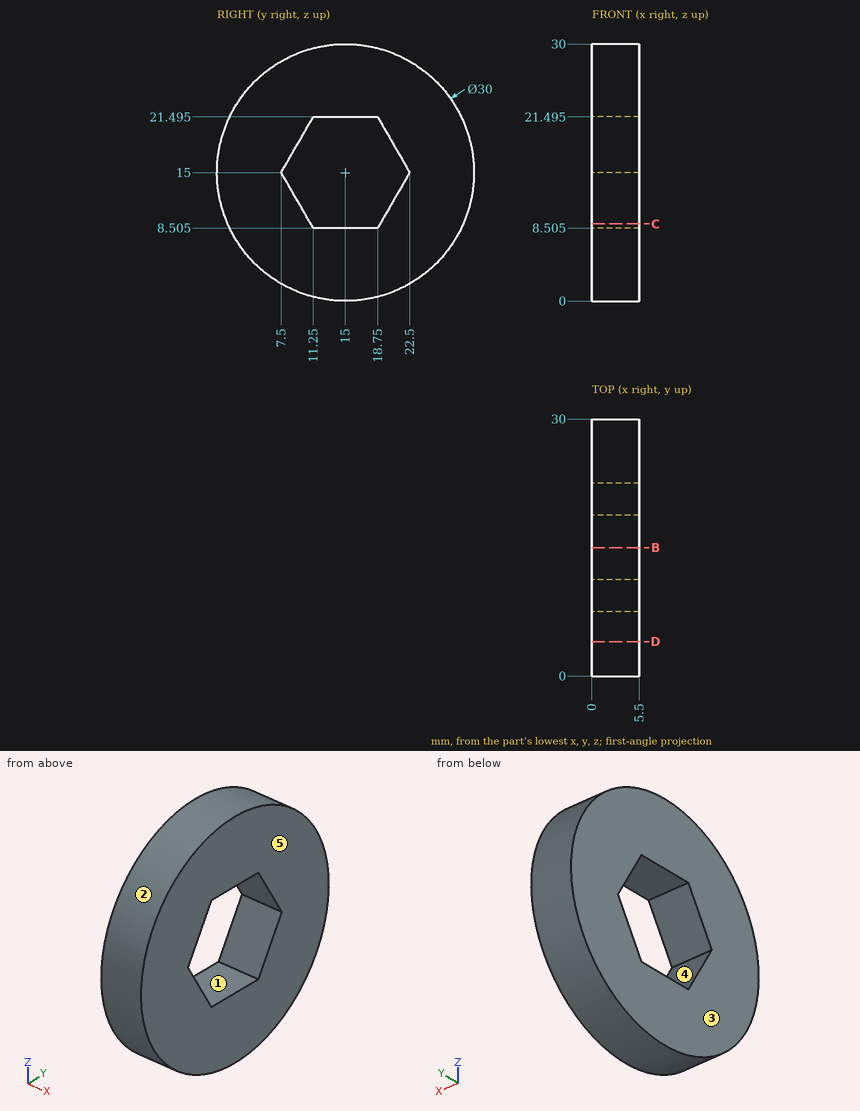
Here's the drawing with two shaded views (mm, measured from the low corner). I have some questions. A direction names the side the tool comes from. Give positions to 0.01 mm unless a question says otherwise; leave off trailing zeros. Order: outer loops, then holes, each group sorted by start corner. A loop starts at its lowest first (then second) coordinate and runs counter-clockwise, first axis right, second up. Notation, with made-up numbers: (29.25, -11.75) - (87.25, -11.75) arc R20 ccw to (87.25, 2.25) - close; hole circle Ø5 at (15.5, 59.5). An arc over 180 degrees is marked (long way). Use a Markdown table: item, result. Add a question column.
Q1. I'm going to push flat-ended pins straight in: pin 1 (2 mm diameter, centred on x = 1, y = 13.5, fed in from +Z); pin 2 (1 mm diameter, centred on x = 1, y = 23, fed in from -Z); pin 3 (2 mm diameter, centred on x = 3, y = 17.5, fed in from +Z) (3 decimals); pin 4 (1.5 mm diameter, centred on y = 18, z = 12, fed in from -X). Where does each tip first touch, or does it pass through?
Q2. If we section it at D-D on y = 4: Write out the boundary of the cut face in (x, z), plus the area to 3 significant figures.
Q3. Please list where these lines run through material, in increasing order: line 1 along Z through (x, y) = (1.65, 12.75) (1 decimal); line 2 along Z through (x, y) = (1.2, 11); line 3 along Y through (x, z) = (2.8, 17.25).
Q4. If we section it at B-B on y = 15: Write out the boundary of the cut face in (x, z) (1 decimal).
Q5. If we section it at C-C on z = 9: Write out the boundary of the cut face in (x, y), plus the area to 3 significant figures.
Q6. On a 3-axis mill with a long thin cutter (end or side, diameter ignored), from which of +Z, -Z, +X, -X, +Y, -Y can I reach the whole of each face in a straight line? I mean the marked faces 4 and 5. Say none if no direction works.
Q7. If we mould it in two halves opening along Z, with no side actions, what happens to the marked faces 1, 2 and 3? For each: released by +Z, released by -Z, zero draft, split by the parting line, or undercut.
Answers follow:
| question | item | result |
|---|---|---|
| 1 | pin 1 | stops at z = 29.99 |
| 1 | pin 2 | stops at z = 2.01 |
| 1 | pin 3 | stops at z = 29.925 |
| 1 | pin 4 | passes through |
| 2 | outline | (0, 4.8) - (5.5, 4.8) - (5.5, 25.2) - (0, 25.2) - close |
| 2 | area | 112 mm^2 |
| 3 | line 1 | z = 0.2 to 8.5, 21.5 to 29.8 |
| 3 | line 2 | z = 0.54 to 8.94, 21.06 to 29.46 |
| 3 | line 3 | y = 0.17 to 8.8, 21.2 to 29.83 |
| 4 | outline | (0, 0) - (5.5, 0) - (5.5, 8.5) - (0, 8.5) - close; (0, 21.5) - (5.5, 21.5) - (5.5, 30) - (0, 30) - close |
| 5 | outline | (0, 1.25) - (5.5, 1.25) - (5.5, 10.96) - (0, 10.96) - close; (0, 19.04) - (5.5, 19.04) - (5.5, 28.75) - (0, 28.75) - close |
| 5 | area | 107 mm^2 |
| 6 | face 4 | +X, -X |
| 6 | face 5 | +Z, -Z, +X, +Y, -Y |
| 7 | face 1 | undercut |
| 7 | face 2 | split by the parting line |
| 7 | face 3 | zero draft |
